Verification items for this drawing (mm, ordinates from the low corner). A direction names the side the tool comes from. Coordinates: 2 decimals unless noted, no trailing zeros. Order: outer loops, then holes, each group sorted by start corner. A loop starts at its lowest first (then second) coordinate and runs counter-clockwise, first axis right, second up.
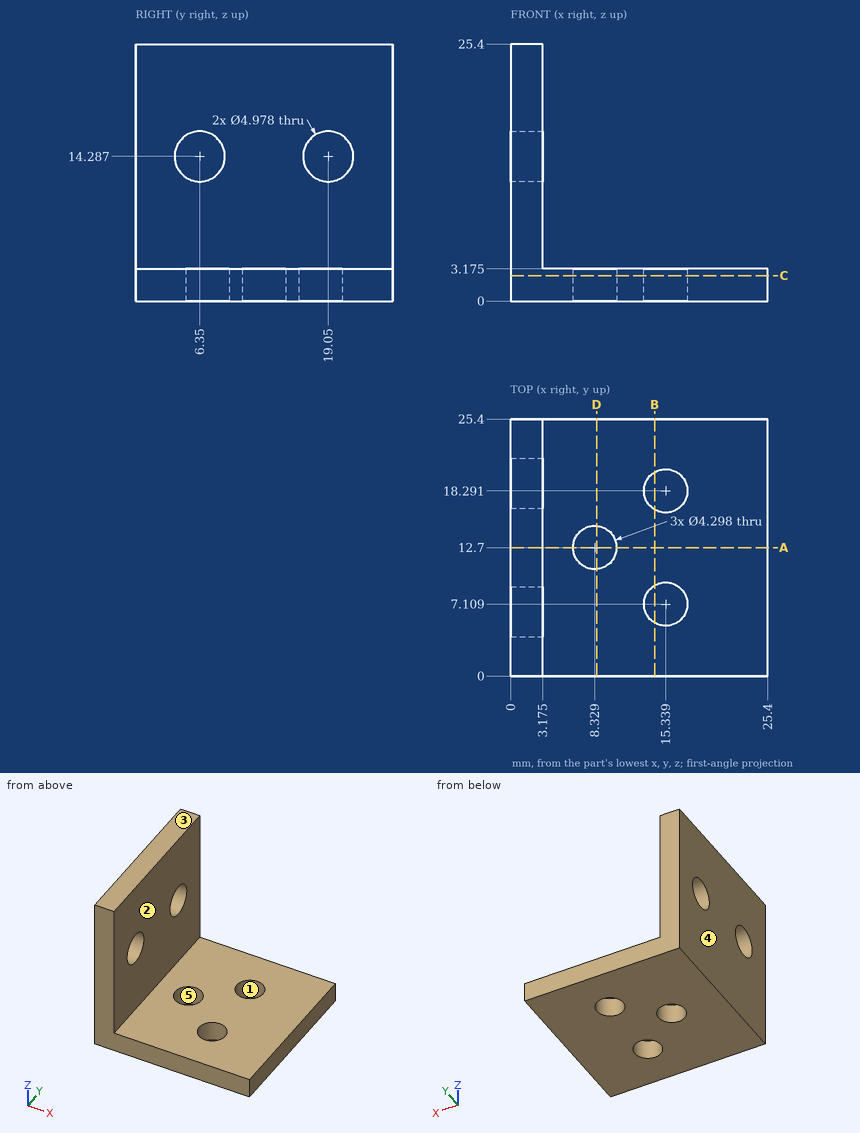
(1) Tool access check on the marked faces 1 and 2. Record the directions out of +Z, -Z, +X, -X, +Y, -Y that give a thin tool (end or side, any length) a straight path to the whole face; none if there is none.
Filled in:
face 1: +Z, -Z
face 2: +Z, +X, +Y, -Y
(2) Cross-section at B-B (x = 14.25). Enter the section's corners in (y, z) (1 decimal).
Filled in:
outline: (0, 0) - (5.3, 0) - (5.3, 3.2) - (0, 3.2) - close; (9, 0) - (16.4, 0) - (16.4, 3.2) - (9, 3.2) - close; (20.1, 0) - (25.4, 0) - (25.4, 3.2) - (20.1, 3.2) - close
(3) Go/stop test with flat-tipped pins: P1, Ø8, axis at x = 10, y = 11.5, coming from the +Z side (1 decimal); P2, Ø2.5, axis at x = 15.34, y = 18.29, coming from the -Z side; P3, Ø6.5, axis at y = 19.05, z = 14.29, coming from the +X side (1 decimal); P4, Ø2, axis at x = 4, z = 3.5, coming from the +Y side. Record where each tip stops, or that it passes through.
Filled in:
P1: stops at z = 3.2
P2: passes through
P3: stops at x = 3.2
P4: stops at y = 25.4
(4) Release check for a two-part mould opening along X. For the marked faces 3, 4 and 5 record: +X half, -X half, draft (parallel to the pull), parting line (faces both ways), or undercut.
Filled in:
face 3: draft
face 4: -X half
face 5: undercut
(5) Cross-section at D-D (x = 8.5). Enter the section's corners in (y, z) (1 decimal).
Filled in:
outline: (0, 0) - (10.6, 0) - (10.6, 3.2) - (0, 3.2) - close; (14.8, 0) - (25.4, 0) - (25.4, 3.2) - (14.8, 3.2) - close
(6) Cross-section at C-C (z = 2.5). Enter the section's corners in (x, y).
Filled in:
outline: (0, 0) - (25.4, 0) - (25.4, 25.4) - (0, 25.4) - close; hole circle Ø4.3 at (8.33, 12.7); hole circle Ø4.3 at (15.34, 7.11); hole circle Ø4.3 at (15.34, 18.29)
(7) Thickness scan on probe 1 along Z at (x, y) = (24, 10) (1 decimal); probe 2 along Y at (x, z) = (7.75, 2.25). Record the ranges inside material, lowest first.
Filled in:
probe 1: z = 0 to 3.2
probe 2: y = 0 to 10.63, 14.77 to 25.4
(8) Cross-section at A-A (y = 12.7). Enter the section's corners in (x, z) (1 decimal).
Filled in:
outline: (0, 0) - (6.2, 0) - (6.2, 3.2) - (3.2, 3.2) - (3.2, 25.4) - (0, 25.4) - close; (10.5, 0) - (25.4, 0) - (25.4, 3.2) - (10.5, 3.2) - close
